```python
from build123d import *

# Parameters (mm, degrees)
F1_DEPTH = 6.35
F2_W     = 6.1722
F2_H     = 25.2222
F3_DEPTH = 25.4


with BuildPart() as f1:
    # F0 (on Top) → F1 (new body)
    with BuildSketch(Plane.XY):
        Polygon((-27.544599, 46.600503), (-53.033499, 46.600503), (-53.033499, 21.111603), (-46.772399, 21.111603), (-46.772399, -4.110597), (-53.033499, -4.110597), (-53.033499, -29.688397), (-46.772399, -29.688397), (-46.772399, -54.910597), (-53.033499, -54.910597), (-53.033499, -80.399497), (-27.544599, -80.399497), (-27.544599, -74.138397), (-2.322399, -74.138397), (-2.322399, -80.399497), (23.255401, -80.399497), (23.255401, -74.138397), (48.477601, -74.138397), (48.477601, -80.399497), (74.055401, -80.399497), (74.055401, -74.138397), (99.277601, -74.138397), (99.277601, -80.399497), (124.766501, -80.399497), (124.766501, -54.910597), (118.505401, -54.910597), (118.505401, -29.688397), (124.766501, -29.688397), (124.766501, -4.110597), (118.505401, -4.110597), (118.505401, 21.111603), (124.766501, 21.111603), (124.766501, 46.600503), (99.277601, 46.600503), (99.277601, 40.339403), (74.055401, 40.339403), (74.055401, 46.600503), (48.477601, 46.600503), (48.477601, 40.339403), (23.255401, 40.339403), (23.255401, 46.600503), (-2.322399, 46.600503), (-2.322399, 40.339403), (-27.544599, 40.339403), align=None)
    extrude(amount=F1_DEPTH)

    # F2 (on face) → F3 (cut)
    with BuildSketch(Plane.XY.offset(6.35)):
        with Locations((35.866501, -42.299497)):
            Rectangle(F2_W, F2_H)
        with Locations((35.866501, 8.500503)):
            Rectangle(F2_W, F2_H)
    extrude(amount=-F3_DEPTH, mode=Mode.SUBTRACT)


solid = f1.part
```
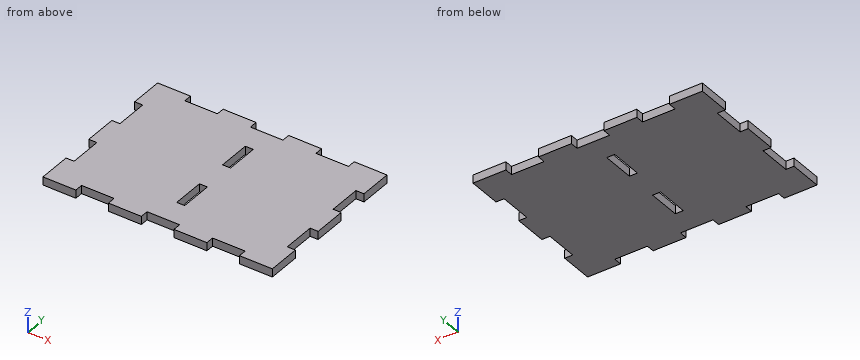
Check sheet for the modelled part. Datum: model origin and axes. Units: mm. Round coordinates to 2 decimals unless told otherwise and drop trailing zeros. Order: outer loops, then holes, each group sorted by start corner. A loop starts at its lowest first (then second) coordinate and runs counter-clockwise, first axis right, second up.
1) Section check B-B (z = 1.5). Give the number of separate pieces and of enclosed holes in the cut face, and give its area (3 significant figures).
2) Go/stop test with flat-tipped pins: pin 1 Ø3 at (y, z) = (-45.5, 3.5) entering from +X; pin 2 Ø3 at (x, z) = (36, 3.5) entering from +Y; pin 3 Ø3 at (x, z) = (36, 4.5) entering from -Y. Record where each tip stops, or that it passes through.
3) Scan lines: line 1 (X direction, y = -39, z = 3); line 2 (X direction, y = 41, z = 5.5); line 3 (Y direction, x = 86, z = 1.5). Record each from-to range of solid material in increasing order.
4) Section check C-C (x = 87.5). Record the boundary of the cut face in (y, z).
5) Section check A-A (y = 6.5). Record the boundary of the cut face in (x, z).
Result:
1. separate pieces: 1
1. enclosed holes: 2
1. area: 20,700 mm2
2. pin 1: stops at x = 118.51
2. pin 2: stops at y = 40.34
2. pin 3: stops at y = -74.14
3. line 1: x = -46.77 to 32.78, 38.95 to 118.51
3. line 2: x = -53.03 to -27.54, -2.32 to 23.26, 48.48 to 74.06, 99.28 to 124.77
3. line 3: y = -74.14 to 40.34
4. outline: (-74.14, 0) - (40.34, 0) - (40.34, 6.35) - (-74.14, 6.35) - close
5. outline: (-46.77, 0) - (32.78, 0) - (32.78, 6.35) - (-46.77, 6.35) - close; (38.95, 0) - (118.51, 0) - (118.51, 6.35) - (38.95, 6.35) - close
